from build123d import *

# Parameters (mm, degrees)
SKETCH5_R   = 3.175
SKETCH5_R_2 = 2.667


with BuildPart() as part:
    # Sweep3: sweep along a curve in space
    with BuildLine() as sweep3_path:
        Line((0, 0, 0), (22.86, 0, 0))
        ThreePointArc((22.86, 0, 0), (31.840256121, 0, -3.719743879), (35.56, 0, -12.7))
        Line((35.56, 0, -12.7), (35.56, 0, -69.48826463))
        ThreePointArc((35.56, 0, -69.48826463), (39.279743879, 0, -78.468520751), (48.26, 0, -82.18826463))
        Line((48.26, 0, -82.18826463), (1483.36, 0, -82.18826463))
    # Sketch5 → Sweep3 (sweep)
    with BuildSketch(Plane(origin=(0, 0, 0), x_dir=(0, 0, -1), z_dir=(1, 0, 0))):
        Circle(SKETCH5_R)
        Circle(SKETCH5_R_2, mode=Mode.SUBTRACT)
    sweep(path=sweep3_path.line)


solid = part.part
The listing builds one solid part. Answer for the finished solid, in the listing's coordinates (mm). Coordinates: 2 decimals unless noted, no trailing zeros. Order: outer loops, then holes, each group sorted by start corner. A loop starts at its lowest first (then second) coordinate and runs counter-clockwise, first axis right, second up.
Q1. Given P1, Ø1, axis at y = 1.5, z = -20, coming from the -X side, flat-ended and moving along its own axis, determine where the tip first touches the part or whether it passes through.
Q2. Consider line 1 (Z direction, x = 650, y = 1); line 2 (Y direction, x = 5, z = 0) (3 decimals); line 3 (X direction, y = -1, z = -56.5). Determine where each line is inside the solid, lowest interval first.
Q3. A cutting plane is placed at A-A, the plane y = 1.5. Write down the section's boundary in (x, z), and give its area (3 significant figures).
Q4. A cutting plane is placed at B-B, the plane z = -50.5. Write down the section's boundary in (x, y) (3 decimals), and give its area (3 significant figures).
Q5. A cutting plane is placed at C-C, the plane x = 441.5. Write down the section's boundary in (y, z) (3 decimals).
Answers follow:
1. P1: stops at x = 32.55
2. line 1: z = -85.2 to -84.66, -79.72 to -79.17
2. line 2: y = -3.175 to -2.667, 2.667 to 3.175
2. line 3: x = 32.55 to 33.09, 38.03 to 38.57
3. outline: (0, -2.8) - (22.86, -2.8) arc R9.9 cw to (32.76, -12.7) - (32.76, -69.49) arc R15.5 ccw to (48.26, -84.99) - (1483.36, -84.99) - (1483.36, -84.39) - (48.26, -84.39) arc R14.91 cw to (33.35, -69.49) - (33.35, -12.7) arc R10.49 ccw to (22.86, -2.21) - (0, -2.21) - close; (0, 2.21) - (22.86, 2.21) arc R14.91 cw to (37.77, -12.7) - (37.77, -69.49) arc R10.49 ccw to (48.26, -79.98) - (1483.36, -79.98) - (1483.36, -79.39) - (48.26, -79.39) arc R9.9 cw to (38.36, -69.49) - (38.36, -12.7) arc R15.5 ccw to (22.86, 2.8) - (0, 2.8) - close
3. area: 1,840 mm2
4. outline: circle Ø6.35 at (35.56, 0); hole circle Ø5.334 at (35.56, 0)
4. area: 9.32 mm2
5. outline: circle Ø6.35 at (0, -82.188); hole circle Ø5.334 at (0, -82.188)
